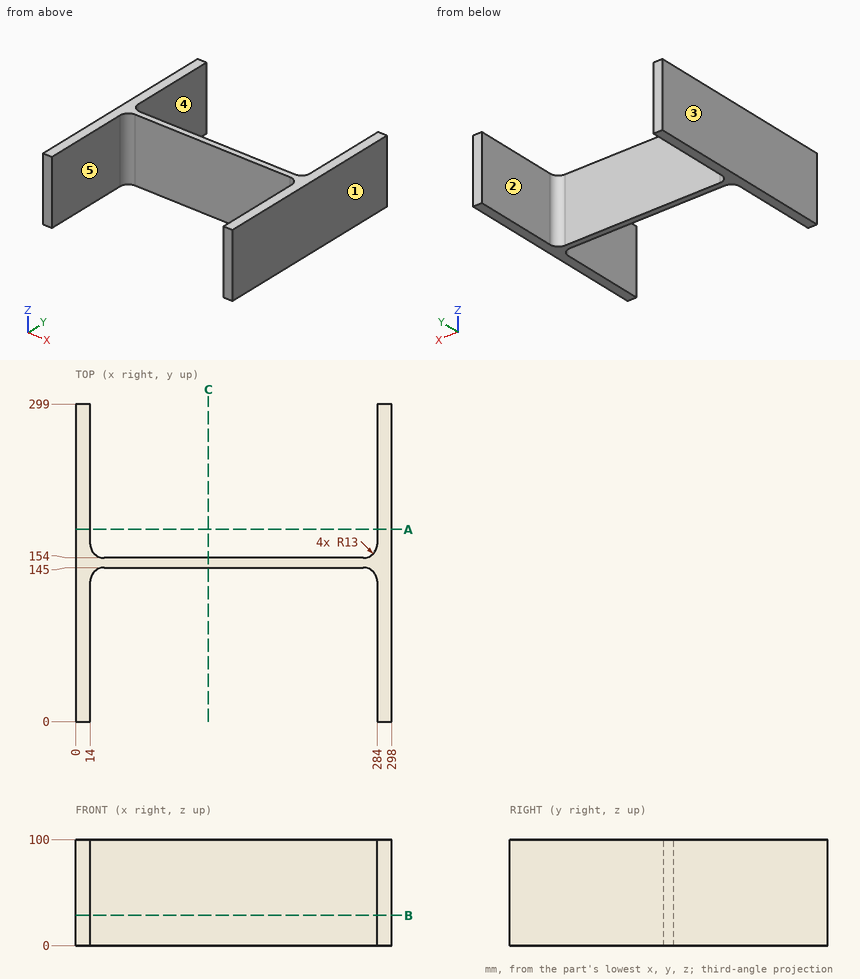
Design review of the part shown in the three views and the two pictorial views. Dimensions are in mm from the part's minimum x, y and z. A direction names the side the tool comes from. Give positions to 0.01 mm unless a question says otherwise; leave off trailing zeros. Write each loop counter-clockwise with the first axis right and the second up, starting at its lowest first coordinate (ties: lowest second). Pieces come first, ordered by that corner, then holes. Notation, with made-up numbers: M 57,-1.5 L 87,-1.5 A12 ccw 87,8.5 Z; hole C -4,-32.75 d10. An arc over 180 degrees is marked long. Answer in a Markdown table with one row per item.
Item 1: Draft analysis for pull direction X (two halves, no side actions). For the marked faces 1, 2 and 3, state which applies: +X half, -X half, draft (parallel to the pull), parting line (faces both ways), or undercut.
Check sheet entries:
| item | result |
|---|---|
| face 1 | +X half |
| face 2 | undercut |
| face 3 | -X half |
Item 2: For P1, Ø10, axis at x = 120.5, z = 25, coming from the -Y side; P2, Ø5, axis at y = 206.5, z = 25.5, coming from the -X side, all flat-tipped, find the tip position at first contact; note any pin that passes through.
Check sheet entries:
| item | result |
|---|---|
| P1 | y = 145 |
| P2 | x = 0 |
Item 3: For line 1 along X through (y, z) = (22, 75); line 2 along Y through (x, z) = (51, 74.5); line 3 along X through (y, z) = (140, 46), list the stretches that pass through material, from the lowest coordinate up.
Check sheet entries:
| item | result |
|---|---|
| line 1 | 0 to 14, 284 to 298 |
| line 2 | 145 to 154 |
| line 3 | 0 to 16.75, 281.25 to 298 |
Item 4: Add section B-B on z = 28.5. Give the boundary of the cut face in (x, y), plus the area to 3 significant figures.
Check sheet entries:
| item | result |
|---|---|
| outline | M 0,0 L 14,0 L 14,132 A13 cw 27,145 L 271,145 A13 cw 284,132 L 284,0 L 298,0 L 298,299 L 284,299 L 284,167 A13 cw 271,154 L 27,154 A13 cw 14,167 L 14,299 L 0,299 Z |
| area | 10,900 mm2 |
Item 5: Tool access review of the marked faces 4 and 5: name each direction out of +Z, -Z, +X, -X, +Y, -Y from which nothing blocks a thin tool from reaching the whole face with its end or side.
Check sheet entries:
| item | result |
|---|---|
| face 4 | +Z, -Z, +Y |
| face 5 | +Z, -Z, -Y |
Item 6: Add section A-A on y = 181. Give the boundary of the cut face in (x, z), plus the area to 3 significant figures.
Check sheet entries:
| item | result |
|---|---|
| outline | M 0,0 L 14,0 L 14,100 L 0,100 Z; M 284,0 L 298,0 L 298,100 L 284,100 Z |
| area | 2,800 mm2 |
Item 7: Add section C-C on x = 125. Give the boundary of the cut face in (y, z).
Check sheet entries:
| item | result |
|---|---|
| outline | M 145,0 L 154,0 L 154,100 L 145,100 Z |
